Autodesk Inventor part; units mm, degrees
ref_plane "YZ Plane" through (0, 0, 0) normal (1, 0, 0) x (0, 1, 0)
ref_plane "XZ Plane" through (0, 0, 0) normal (0, 1, 0) x (-1, 0, 0)
ref_plane "XY Plane" through (0, 0, 0) normal (0, 0, 1) x (1, 0, 0)
sketch "Sketch1" plane through (0, 0, 0) normal (0, 1, 0) x (-1, 0, 0)
  circle A0 centre (146.7383, -31.3394) radius 6.1
  circle A1 centre (146.7383, -31.3394) radius 7.5
  circle A2 centre (-107.7617, -44.8394) radius 7.5
  circle A3 centre (-107.7617, -44.8394) radius 6
  circle A4 centre (-142.7617, -335.2394) radius 7.5
  circle A5 centre (-142.7617, -335.2394) radius 6
  circle A6 centre (-314.7617, -335.1394) radius 7.5
  circle A7 centre (-314.7617, -335.1394) radius 6.1
  circle A8 centre (-322.7617, -31.3394) radius 7.5
  circle A9 centre (-322.7617, -31.3394) radius 6.1
  line L0 (-322.7617, -23.8394) -> (146.7383, -23.8394)
  line L1 (146.7383, -38.8394) -> (-107.7617, -38.8394)
  line L2 (-107.7587, -37.3394) -> (146.7359, -37.4394)
  line L3 (146.7383, -25.2394) -> (-322.7617, -25.2394)
  line L4 (-328.8595, -31.5) -> (-320.8595, -335.3)
  line L5 (-322.2591, -335.3369) -> (-330.2591, -31.5369)
  line L6 (-314.7617, -341.2394) -> (-142.7617, -341.2394)
  line L7 (-142.766, -342.7394) -> (-314.766, -342.6394)
  line L8 (-115.2617, -44.8394) -> (-115.2617, -185.0394)
  line L9 (-115.2617, -185.0394) -> (-113.7617, -185.0394)
  line L10 (-113.7617, -185.0394) -> (-113.7617, -44.8394)
  line L11 (-136.7617, -335.2394) -> (-136.7617, -195.0394)
  line L12 (-136.7617, -195.0394) -> (-135.2617, -195.0394)
  line L13 (-135.2617, -195.0394) -> (-135.2617, -335.2394)
  arc A10 (-100.7617, -192.5394) -> (-100.7617, -187.5394) centre (-96.4315, -190.0394) ccw
  point P0 (0, 0)
  point P1 (-147.2617, -341.2394)
extrude "Extrusion1" add sketch "Sketch1" against normal blind 6 contours A0 L3 A1 L2 | L3 A8 L0 A1 | A1 L1 A2 L2 | L3 A9 L4 A8 | A2 L1 A3 L10 | A2 L10 L9 L8 | A8 L4 A6 L5 | A6 L4 A7 L6 | A6 L6 A4 L7 | A4 L6 A5 L11 | A4 L11 L12 L13 picked at (144.276, -37.6941) picked at (-329.0502, -33.966) picked at (-114.0352, -47.3793) picked at (-312.3021, -341.4951) picked at (-136.4882, -332.6995)
properties part number "Belt_1" material "Rubber"
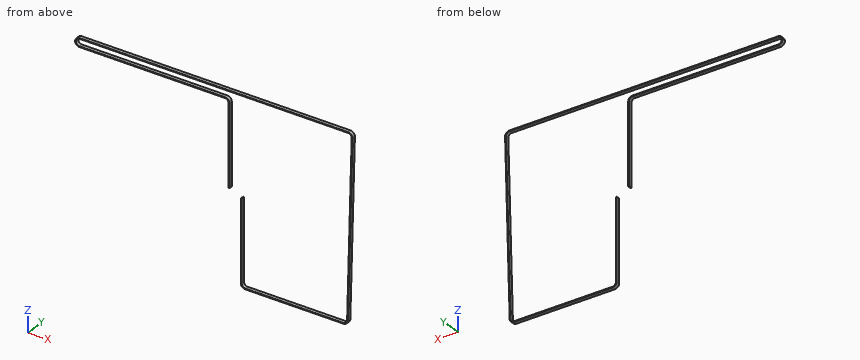
Here's how the part is built. I have some questions about the finished solid (model axes, mm). Give positions to 0.01 mm unless a question says otherwise; leave off trailing zeros. Loops run counter-clockwise (first coordinate to the right, second up) from the corner with the lowest first, then second, coordinate; pieces in that order, holes last. Notation, with made-up numbers: (84.5, 73.25) -> (140.5, 73.25) arc R18 cw to (140.5, 108.25) -> close; hole circle Ø1 at (9.5, 39.5). An arc over 180 degrees is marked (long way). Answer as a JSON object with one key per item and string values. Group by question number.
Item 1: Imagine slicing it at C-C on y = -1.7. Write out the boundary of the cut face in (x, z), then the cut area to 3 significant figures.
Item 2: Imagine slicing it at A-A on x = 204. Write out the boundary of the cut face in (y, z).
Item 3: I need wall thicknesses on L1, parallel to Z at x = 15.5, y = -1.5; L2, parallel to Z at x = 250.5, y = -4.85; L3, parallel to X at y = -5.25, z = -57. Which ranges of each line are inside material? Lowest first, please.
Item 4: Imagine slicing it at B-B on z = -203. Write out the boundary of the cut face in (x, y), then the cut area to 3 significant figures.
Item 5: Will these pins go through, and if not, where does the flat tip stop? pin 1 (2 mm diameter, centred on x = 62.5, y = -4, fed in from -Z); pin 2 (3 mm diameter, centred on y = -3.5, z = -263.5, fed in from +X); pin 3 (3 mm diameter, centred on y = -4.5, z = -267.5, fed in from -X).
Answer list:
{
 "1": {"outline": "(-146.74, -38.84) -> (107.76, -38.84) arc R6 cw to (113.76, -44.84) -> (113.76, -185.04) -> (115.26, -185.04) -> (115.26, -44.84) arc R7.5 ccw to (107.76, -37.34) -> (-146.74, -37.44) arc R6.1 cw to (-146.74, -25.24) -> (322.76, -25.24) arc R6.1 cw to (328.86, -31.5) -> (320.86, -335.3) arc R6.1 cw to (314.76, -341.24) -> (142.76, -341.24) arc R6 cw to (136.76, -335.24) -> (136.76, -195.04) -> (135.26, -195.04) -> (135.26, -335.24) arc R7.5 ccw to (142.77, -342.74) -> (314.77, -342.64) arc R7.5 ccw to (322.26, -335.34) -> (330.26, -31.54) arc R7.5 ccw to (322.76, -23.84) -> (-146.74, -23.84) arc R7.5 ccw to start", "area": "2,210 mm2"},
 "2": {"outline": "(-6, -342.7) -> (0, -342.7) -> (0, -341.24) -> (-6, -341.24) -> close; (-6, -25.24) -> (0, -25.24) -> (0, -23.84) -> (-6, -23.84) -> close"},
 "3": {"L1": "z = -38.84 to -37.38, -25.24 to -23.84", "L2": "z = -342.68 to -341.24, -25.24 to -23.84", "L3": "x = 113.76 to 115.26, 328.19 to 329.59"},
 "4": {"outline": "(135.26, -6) -> (136.76, -6) -> (136.76, 0) -> (135.26, 0) -> close; (324.34, -6) -> (325.74, -6) -> (325.74, 0) -> (324.34, 0) -> close", "area": "17.4 mm2"},
 "5": {"pin 1": "stops at z = -38.84", "pin 2": "stops at x = 324.19", "pin 3": "stops at x = 135.26"}
}
